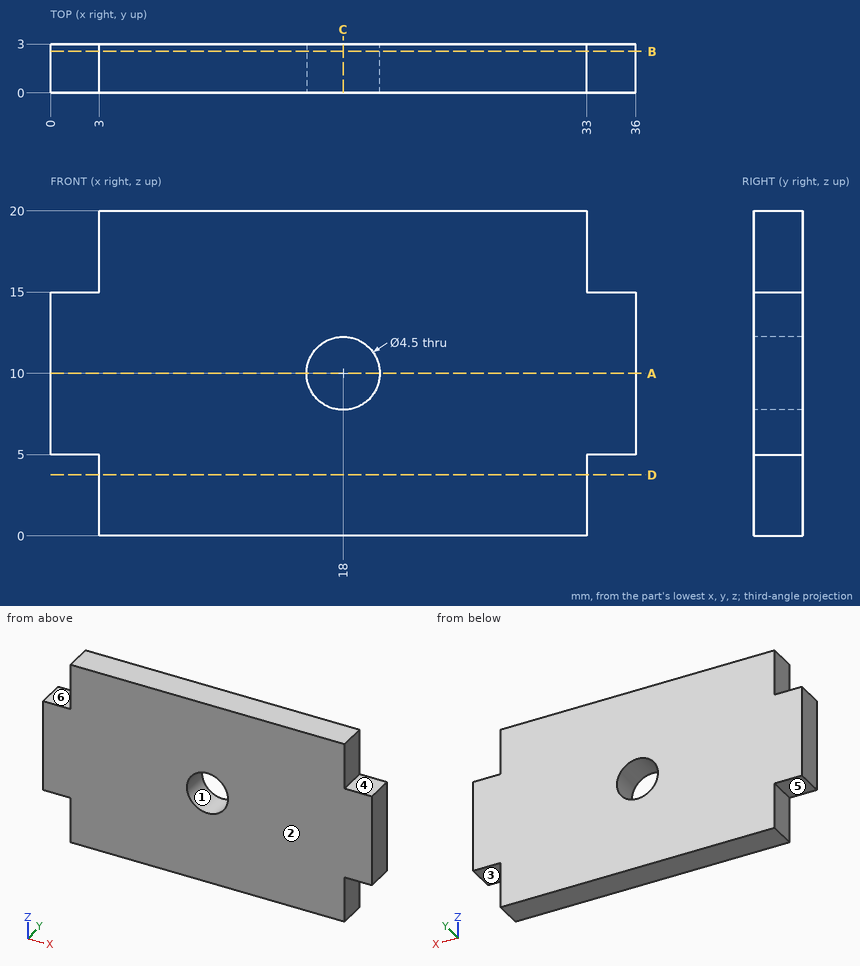
Geometry check sheet. Reference: drawing and pictorial views, mm from the part's lowest x, y, z. A direction names the side the tool comes from. Round coordinates to 2 decimals unless told otherwise and drop trailing zeros. Write each loop counter-clockwise with the first axis right and the second up, starting at its lowest first coordinate (ties: lowest second). Pieces come first, ordered by that corner, then holes.
(1) Section check A-A (z = 10). Enter the section's corners in (x, y).
Returned:
outline: (0, 0) - (15.75, 0) - (15.75, 3) - (0, 3) - close; (20.25, 0) - (36, 0) - (36, 3) - (20.25, 3) - close
(2) Material ranges on line 1 (X direction, y = 1.65, z = 10); line 2 (Z direction, x = 18, y = 2.25); line 3 (X direction, y = 0.95, z = 16.5), recorded low to high.
Returned:
line 1: x = 0 to 15.75, 20.25 to 36
line 2: z = 0 to 7.75, 12.25 to 20
line 3: x = 3 to 33
(3) Depth check by flat-ended pin: pin 1 Ø2 at (x, z) = (21.5, 11.5) entering from -Y; pin 2 Ø0.9 at (x, y) = (1.5, 1) entering from -Z; pin 3 Ø0.9 at (x, y) = (35, 1.5) entering from +Z; pin 4 Ø1.5 at (y, z) = (2, 18) entering from -X. Enter the tip coordinate at first touch or a pass-through.
Returned:
pin 1: stops at y = 0
pin 2: stops at z = 5
pin 3: stops at z = 15
pin 4: stops at x = 3
(4) Access from +Z, -Z, +X, -X, +Y, -Y to the whole of each face (thin tool, end or side, straight path). Record for the marked faces 3, 4, 5 and 6.
Returned:
face 3: -Z, +X, +Y, -Y
face 4: +Z, +X, +Y, -Y
face 5: -Z, -X, +Y, -Y
face 6: +Z, -X, +Y, -Y
(5) Mould release check, pull along X, two halves, no side actions. Record for the marked faces 1 and 2: pulls with the +X half, pulls with the -X half, needs draft (parallel to the pull), parting line crosses it, or undercut.
Returned:
face 1: undercut
face 2: needs draft
(6) Section check C-C (x = 18). Enter the section's corners in (y, z).
Returned:
outline: (0, 0) - (3, 0) - (3, 7.75) - (0, 7.75) - close; (0, 12.25) - (3, 12.25) - (3, 20) - (0, 20) - close
(7) Section check D-D (z = 3.75). Enter the section's corners in (x, y), plus the area to 3 significant figures.
Returned:
outline: (3, 0) - (33, 0) - (33, 3) - (3, 3) - close
area: 90.0 mm2
(8) Section check B-B (y = 2.55). Enter the section's corners in (x, z), plus the area to 3 significant figures.
Returned:
outline: (0, 5) - (3, 5) - (3, 0) - (33, 0) - (33, 5) - (36, 5) - (36, 15) - (33, 15) - (33, 20) - (3, 20) - (3, 15) - (0, 15) - close; hole circle Ø4.5 at (18, 10)
area: 644 mm2
